Part model, mm, in its own coordinate system. Coordinates: 2 decimals unless noted, no trailing zeros. Loops run counter-clockwise (first coordinate to the right, second up) from the corner with the lowest first, then second, coordinate; pieces in that order, holes last.
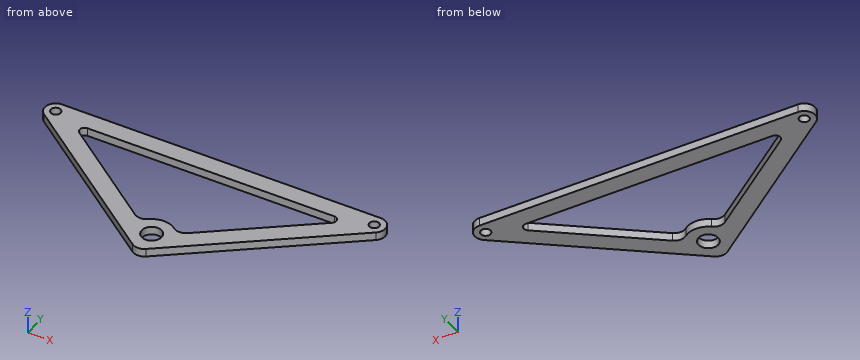
```python
from build123d import *

# Parameters (mm, degrees)
SKETCH1_R           = 3
SKETCH1_R_2         = 6
BOSS_EXTRUDE1_DEPTH = 2.5


with BuildPart() as part:
    # Sketch1 → Boss-Extrude1 (new body, symmetric)
    with BuildSketch(Plane.XY):
        with BuildLine():
            Line((96.909065007, 0), (-96.909065007, 0))
            ThreePointArc((-96.909065007, 0), (-103.256738035, -4.565267366), (-100.94836092, -12.035609666))
            Line((-100.94836092, -12.035609666), (-4.039295913, -85.339986595))
            ThreePointArc((-4.039295913, -85.339986595), (0, -86.695623071), (4.039295913, -85.339986595))
            Line((4.039295913, -85.339986595), (100.94836092, -12.035609666))
            ThreePointArc((100.94836092, -12.035609666), (103.256738035, -4.565267366), (96.909065007, 0))
        make_face()
        with Locations((96.909065007, -6.695623071)):
            Circle(SKETCH1_R, mode=Mode.SUBTRACT)
        with Locations((-96.909065007, -6.695623071)):
            Circle(SKETCH1_R, mode=Mode.SUBTRACT)
        with Locations((0, -72.476809125)):
            Circle(SKETCH1_R_2, mode=Mode.SUBTRACT)
        with BuildLine():
            Line((-76.954542332, -16.392601796), (-15.971447816, -62.521699692))
            ThreePointArc((-15.971447816, -62.521699692), (-11.880304954, -63.878041653), (-7.809525514, -62.461754894))
            ThreePointArc((-7.809525514, -62.461754894), (0, -59.776809125), (7.809525514, -62.461754894))
            ThreePointArc((7.809525514, -62.461754894), (11.880304954, -63.878041653), (15.971447816, -62.521699692))
            Line((15.971447816, -62.521699692), (76.954542332, -16.392601796))
            ThreePointArc((76.954542332, -16.392601796), (77.988819691, -13.045485827), (75.144720063, -11))
            Line((75.144720063, -11), (-75.144720063, -11))
            ThreePointArc((-75.144720063, -11), (-77.988819691, -13.045485827), (-76.954542332, -16.392601796))
        make_face(mode=Mode.SUBTRACT)
    extrude(amount=BOSS_EXTRUDE1_DEPTH, both=True)


solid = part.part
```
Q1. Probe line 1 (Y direction, x = -4.5, z = -1.9); line 2 (Y direction, x = 0, z = -0.95); line 3 (X direction, y = -48.5, z = -1.75). List the from-to ranges inside material, lowest first.
Q2. Saw through at A-A (x = 0). List the corners of the cut face in (y, z).
Q3. Saw through at C-C (x = -59.5). List the corners of the cut face in (y, z), plus the area to 3 significant figures.
Q4. Saw through at B-B (y = -24.5). List the corners of the cut face in (x, z), plus the area to 3 significant figures.
Q5. Saw through at D-D (z = 0.85). List the corners of the cut face in (x, y), plus the area to 3 significant figures.
Checked values:
1. line 1: y = -84.99 to -76.45, -68.51 to -60.6, -11 to 0
1. line 2: y = -86.7 to -78.48, -66.48 to -59.78, -11 to 0
1. line 3: x = -52.74 to -34.51, 34.51 to 52.74
2. outline: (-86.7, -2.5) - (-78.48, -2.5) - (-78.48, 2.5) - (-86.7, 2.5) - close; (-66.48, -2.5) - (-59.78, -2.5) - (-59.78, 2.5) - (-66.48, 2.5) - close; (-11, -2.5) - (0, -2.5) - (0, 2.5) - (-11, 2.5) - close
3. outline: (-43.39, -2.5) - (-29.6, -2.5) - (-29.6, 2.5) - (-43.39, 2.5) - close; (-11, -2.5) - (0, -2.5) - (0, 2.5) - (-11, 2.5) - close
3. area: 124 mm2
4. outline: (-84.47, -2.5) - (-66.24, -2.5) - (-66.24, 2.5) - (-84.47, 2.5) - close; (66.24, -2.5) - (84.47, -2.5) - (84.47, 2.5) - (66.24, 2.5) - close
4. area: 182 mm2
5. outline: (-100.95, -12.04) - (-4.04, -85.34) arc R6.7 ccw to (4.04, -85.34) - (100.95, -12.04) arc R6.7 ccw to (96.91, 0) - (-96.91, 0) arc R6.7 ccw to start; hole circle Ø6 at (-96.91, -6.7); hole (-76.95, -16.39) - (-15.97, -62.52) arc R6.7 ccw to (-7.81, -62.46) arc R12.7 cw to (7.81, -62.46) arc R6.7 ccw to (15.97, -62.52) - (76.95, -16.39) arc R3 ccw to (75.14, -11) - (-75.14, -11) arc R3 ccw to start; hole circle Ø12 at (0, -72.48); hole circle Ø6 at (96.91, -6.7)
5. area: 4,890 mm2
